Build history of the part. All positions in model axes, mm. Give positions to 0.01 mm unless a question says otherwise; leave off trailing zeros. Write each loop counter-clockwise with the first axis right and the second up, starting at its lowest first coordinate (ties: lowest second). Pieces come first, ordered by that corner, then holes. Notation, with made-up numbers: (-32, 55) -> (5, 55) arc R14 cw to (5, 78) -> close; hole circle Ø5 at (-4.75, 51). An arc over 180 degrees is marked (long way). Put each result on its own line as item: value. Start each with the question number.
Item 1: Slice it at A-A, the plane z = 1.2. List the corners of the cut face in (x, y), plus the area to 3 significant figures.
Item 2: Slice it at B-B, the plane y = 248.5. List the corners of the cut face in (x, z), plus the area to 3 significant figures.
Item 3: Slice it at D-D, the plane x = -26. List the corners of the cut face in (y, z), plus the area to 3 significant figures.
Item 4: Slice it at C-C, the plane x = -269.5. List the corners of the cut face in (y, z), plus the area to 3 significant figures.
Item 5: Drill centre lines: line 1 along Y through (x, z) = (-258, 1.4); line 2 along X through (y, z) = (230.5, 3.95); line 3 along Y through (x, z) = (-351, 1.5). Where is each one in solid material? Low to high.
Item 6: Flat gauge pins, fed straight in: pin 1 Ø1.8 at (y, z) = (251, 3) entering from -X; pin 2 Ø1.8 at (y, z) = (254, 4) entering from +X; pin 3 Ø5 at (x, y) = (-155, 213) entering from -Z; pin 4 Ø1 at (x, z) = (-251.5, 1) entering from +Y. Where does each tip first touch, or does it go through?
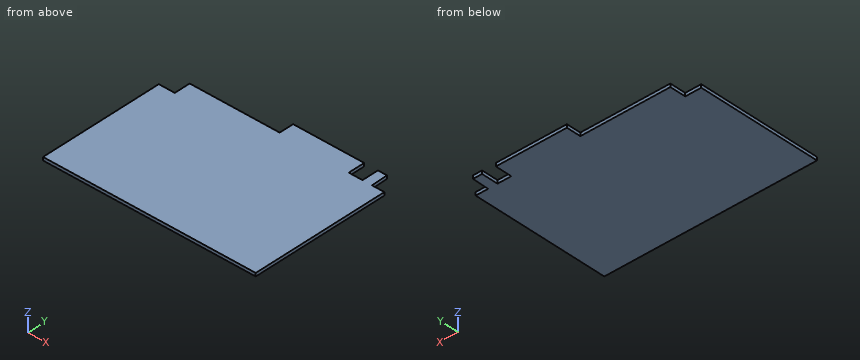
```python
from build123d import *

# Parameters (mm, degrees)
BOSS_EXTRUDE1_DEPTH = 6
SKETCH2_W           = 30
SKETCH2_H           = 30
CUT_EXTRUDE1_DEPTH  = 10
SKETCH3_W           = 398.694966145
SKETCH3_H           = 1
CUT_EXTRUDE2_DEPTH  = 10


with BuildPart() as part:
    # Sketch1 → Boss-Extrude1 (new body)
    with BuildSketch(Plane.XY):
        Polygon((28.571428571, 236.060202245), (28.571428571, 237.05184048), (5.415486436, 237.05184048), (4.571428571, 268.104761905), (-12.428571429, 268.104761905), (-12.428571429, 237.05184048), (-38.216595912, 237.05184048), (-38.216595912, 268.104761905), (-171.428571429, 268.104761905), (-171.428571429, 241.104761905), (-370.123537574, 241.104761905), (-370.123537574, -22.895238095), (28.571428571, -22.895238095), align=None)
    extrude(amount=BOSS_EXTRUDE1_DEPTH)

    # Sketch2 → Cut-Extrude1 (cut)
    with BuildSketch(Plane.XY.offset(6)):
        with Locations((-355.123537574, 226.104761905)):
            Rectangle(SKETCH2_W, SKETCH2_H)
    extrude(amount=-CUT_EXTRUDE1_DEPTH, mode=Mode.SUBTRACT)

    # Sketch3 → Cut-Extrude2 (cut)
    with BuildSketch(Plane.XY.offset(6)):
        with Locations((-170.776054501, -22.395238095)):
            Rectangle(SKETCH3_W, SKETCH3_H)
    extrude(amount=-CUT_EXTRUDE2_DEPTH, mode=Mode.SUBTRACT)


solid = part.part
```
Values follow:
1. outline: (-370.12, -21.9) -> (28.57, -21.9) -> (28.57, 237.05) -> (5.42, 237.05) -> (4.57, 268.1) -> (-12.43, 268.1) -> (-12.43, 237.05) -> (-38.22, 237.05) -> (-38.22, 268.1) -> (-171.43, 268.1) -> (-171.43, 241.1) -> (-340.12, 241.1) -> (-340.12, 211.1) -> (-370.12, 211.1) -> close
1. area: 108,000 mm2
2. outline: (-171.43, 0) -> (-38.22, 0) -> (-38.22, 6) -> (-171.43, 6) -> close; (-12.43, 0) -> (5.1, 0) -> (5.1, 6) -> (-12.43, 6) -> close
2. area: 904 mm2
3. outline: (-21.9, 0) -> (237.05, 0) -> (237.05, 6) -> (-21.9, 6) -> close
3. area: 1,550 mm2
4. outline: (-21.9, 0) -> (241.1, 0) -> (241.1, 6) -> (-21.9, 6) -> close
4. area: 1,580 mm2
5. line 1: -21.9 to 241.1
5. line 2: -340.12 to 28.57
5. line 3: -21.9 to 211.1
6. pin 1: x = -171.43
6. pin 2: x = 4.98
6. pin 3: z = 0
6. pin 4: y = 241.1
